The drawing under review shows one solid part. Ordinate dimensions are in mm from its lowest x, y, z. A direction names the side the tool comes from. Coordinates: 2 decimals unless noted, no trailing zeros. Order: outer loops, then holes, each group sorted by start corner. A loop starts at its lowest first (then second) coordinate and runs counter-clockwise, first axis right, second up. Notation, with made-up numbers: (-16, -12.75) -> (16, -12.75) arc R17 ccw to (16, -3.75) -> close; hole circle Ø6 at (-34.75, 44). An arc over 180 degrees is marked (long way). Use a Markdown table: item, result. Add a question column.
Q1. Add section B-B (x = 10.75). State the section outline as (y, z) points.
Q2. Add section C-C (y = 38). State the section outline as (x, z) points, then the cut area to 3 significant figures.
Q3. Machinability: for the marked faces 4 and 5, which of the approach directions +Z, -Z, +X, -X, +Y, -Y give a long, thin tool a straight path to every point of the face, cutting with its end or side? Answer none if there is none.
Q4. The part is to be moulded in two halves that separate along Y. For the marked faces 1, 2 and 3, say which applies: pulls with the +Y half, pulls with the -Y half, needs draft (parallel to the pull), parting line crosses it, or undercut.
Q5. Add section A-A (z = 48). State the section outline as (x, y) points, then the cut area to 3 significant figures.
Q6. Wall thickness on probe 1 along Y at (x, z) = (10.5, 13.5); probe 2 along Z at (x, y) = (1.5, 50.5): over which ranges is each line inside the solid? List them lowest first.
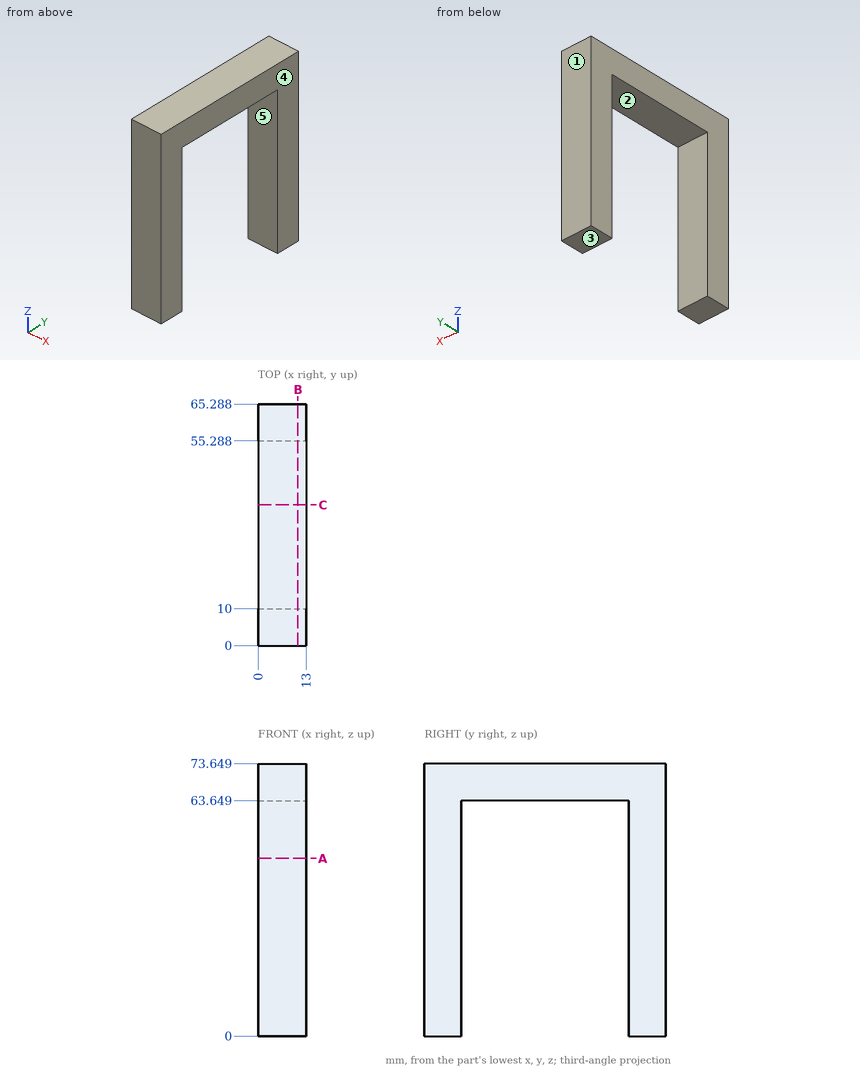
Established:
| question | item | result |
|---|---|---|
| 1 | outline | (0, 0) -> (10, 0) -> (10, 63.65) -> (55.29, 63.65) -> (55.29, 0) -> (65.29, 0) -> (65.29, 73.65) -> (0, 73.65) -> close |
| 2 | outline | (0, 63.65) -> (13, 63.65) -> (13, 73.65) -> (0, 73.65) -> close |
| 2 | area | 130 mm^2 |
| 3 | face 4 | +Z, -Z, +X, +Y, -Y |
| 3 | face 5 | -Z, +X, -X |
| 4 | face 1 | pulls with the +Y half |
| 4 | face 2 | undercut |
| 4 | face 3 | needs draft |
| 5 | outline | (0, 0) -> (13, 0) -> (13, 10) -> (0, 10) -> close; (0, 55.29) -> (13, 55.29) -> (13, 65.29) -> (0, 65.29) -> close |
| 5 | area | 260 mm^2 |
| 6 | probe 1 | 0 to 10, 55.29 to 65.29 |
| 6 | probe 2 | 63.65 to 73.65 |
